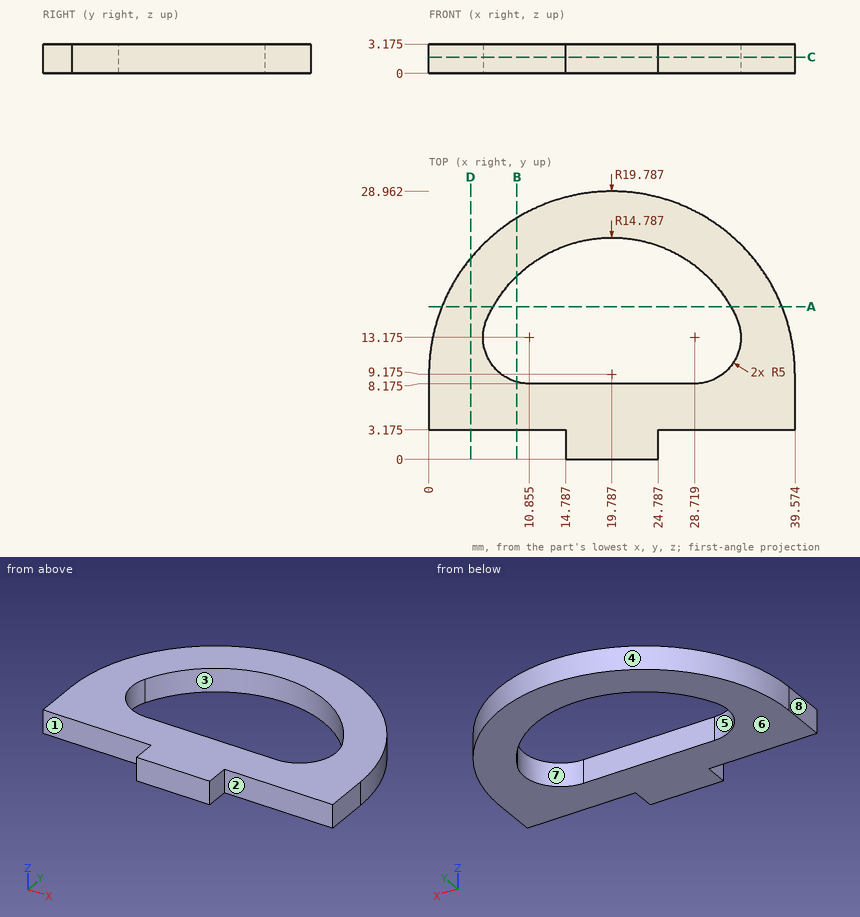
Here's the drawing with two shaded views (mm, measured from the low corner). I have some questions. A direction names the side the tool comes from. Coordinates: 2 decimals unless noted, no trailing zeros. Order: outer loops, then holes, each group sorted by start corner. A loop starts at its lowest first (then second) coordinate and runs counter-clockwise, first axis right, second up.
Item 1: If we section it at A-A, the plane y = 16.5: List the corners of the cut face in (x, z) for me (1 decimal).
Response values:
outline: (1.4, 0) - (6.9, 0) - (6.9, 3.2) - (1.4, 3.2) - close; (32.6, 0) - (38.2, 0) - (38.2, 3.2) - (32.6, 3.2) - close
Item 2: If we section it at D-D, the plane x = 4.5: List the corners of the cut face in (y, z) for me (1 decimal).
Response values:
outline: (3.2, 0) - (21.7, 0) - (21.7, 3.2) - (3.2, 3.2) - close
Item 3: Which directions (+Z, -Z, +X, -X, +Y, -Y) give clear straight access to the entire face, cutting with the end or side of a thin tool? Please do the marked faces 1, 2, 3 and 4.
Response values:
face 1: +Z, -Z, -X, -Y
face 2: +Z, -Z, +X, -Y
face 3: +Z, -Z
face 4: +Z, -Z, +Y
Item 4: If we section it at B-B, the plane x = 9.5: List the corners of the cut face in (y, z) for me (1 decimal).
Response values:
outline: (3.2, 0) - (8.4, 0) - (8.4, 3.2) - (3.2, 3.2) - close; (19.8, 0) - (26.1, 0) - (26.1, 3.2) - (19.8, 3.2) - close
Item 5: Thinking about a two-plate mould opening in X: for the marked faces 5, 6, 7 and 8, which applies, pulls with the +X half, pulls with the -X half, needs draft (parallel to the pull), parting line crosses it, or undercut?
Response values:
face 5: undercut
face 6: needs draft
face 7: undercut
face 8: pulls with the -X half
Item 6: I need wall thicknesses on probe 1 along X at (y, z) = (17.75, 0.2) (1 decimal); probe 2 along X at (y, z) = (3, 1.2); probe 3 along X at (y, z) = (21.5, 2) (1 decimal). Which ranges of each line are inside material? Lowest first, please.
Response values:
probe 1: x = 2 to 7.7, 31.8 to 37.6
probe 2: x = 14.79 to 24.79
probe 3: x = 4.3 to 11.6, 28 to 35.3
Item 7: I'm going to push flat-ended pins straight in: pin 1 Ø1 at (y, z) = (14, 1) entering from -X; pin 2 Ø1.6 at (x, z) = (34.5, 2) entering from -Y (3 decimals); pin 3 Ø1.6 at (x, z) = (18, 1) entering from +Y. Where does each tip first touch, or does it pass through?
Response values:
pin 1: stops at x = 0.48
pin 2: stops at y = 3.175
pin 3: stops at y = 28.94
Item 8: If we section it at C-C, the plane z = 1.75: List the corners of the cut face in (x, y) for me (1 decimal).
Response values:
outline: (0, 3.2) - (14.8, 3.2) - (14.8, 0) - (24.8, 0) - (24.8, 3.2) - (39.6, 3.2) - (39.6, 9.2) arc R19.8 ccw to (0, 9.2) - close; hole (6.3, 15.2) arc R5 ccw to (10.9, 8.2) - (28.7, 8.2) arc R5 ccw to (33.3, 15.2) arc R14.8 ccw to start
